Check sheet for the modelled part. Datum: model origin and axes. Units: mm. A direction names the side the tool comes from. Round coordinates to 2 decimals unless told otherwise and drop trailing zeros. Loops run counter-clockwise (first coordinate to the right, second up) from the corner with the lowest first, then second, coordinate; pieces in that order, holes last. Notation, with made-up numbers: (22, 86) - (64, 86) arc R32 cw to (64, 125) - close; hole circle Ø8 at (24.25, 84.5). An arc over 180 degrees is marked (long way). Put each result on its own line as item: value. Start each with the question number.
Autodesk Inventor part; units mm, degrees
ref_plane "YZ Plane" through (0, 0, 0) normal (1, 0, 0) x (0, 1, 0)
ref_plane "XZ Plane" through (0, 0, 0) normal (0, 1, 0) x (-1, 0, 0)
ref_plane "XY Plane" through (0, 0, 0) normal (0, 0, 1) x (1, 0, 0)
sketch "Sketch1" plane through (0, 0, 0) normal (0, 0, 1) x (1, 0, 0)
  line L0 (29.7558, 35.4616) -> (45.5886, 8.0385)
  line L1 (45.5886, 8.0385) -> (40.0899, -23.1459)
  line L2 (40.0899, -23.1459) -> (15.8328, -43.5001)
  line L3 (15.8328, -43.5001) -> (-15.8328, -43.5001)
  line L4 (-15.8328, -43.5001) -> (-40.0899, -23.1459)
  line L5 (-40.0899, -23.1459) -> (-45.5886, 8.0385)
  line L6 (-45.5886, 8.0385) -> (-29.7558, 35.4616)
  line L7 (-29.7558, 35.4616) -> (0, 46.2919)
  line L8 (0, 46.2919) -> (29.7558, 35.4616)
  line L9 (-29.7558, 35.4616) -> (0, 87.0003)
  line L10 (0, 87.0003) -> (29.7558, 35.4616)
  line L11 (0, 93.0003) -> (-48.7326, 8.5929)
  line L12 (-48.7326, 8.5929) -> (-42.8548, -24.7422)
  line L13 (-42.8548, -24.7422) -> (-16.9247, -46.5001)
  line L14 (-16.9247, -46.5001) -> (16.9247, -46.5001)
  line L15 (16.9247, -46.5001) -> (42.8548, -24.7422)
  line L16 (42.8548, -24.7422) -> (48.7326, 8.5929)
  line L17 (48.7326, 8.5929) -> (0, 93.0003)
  line L18 (0, -74.4002) -> (0, 120.9003)
  point P0 (0, 0)
  point P1 (0, 0)
  dimension "d0" = 89.792
  dimension "d1" = 3
  dimension "d2" = 3
  dimension "d3" = 3
  dimension "d4" = 3
extrude "Extrusion1" add sketch "Sketch1" along normal mid plane 20 contours L10 L18 L17 L16 L15 L14 L3 L2 L1 L0 | L9 L6 L5 L4 L3 L18 L14 L13 L12 L11
sketch "Sketch2" plane through (0, 0, 10) normal (0, 0, 1) x (1, 0, 0)
  line L0 (-1.5, 90.4022) -> (-1.5, 84.4022)
  line L1 (0, 87.0003) -> (-45.5886, 8.0385)
  line L2 (45.5886, 8.0385) -> (0, 87.0003)
  line L3 (1.5, 84.4022) -> (1.5, 90.4022)
  line L4 (48.7326, 8.5929) -> (0, 93.0003)
  line L5 (16.9247, -46.5001) -> (42.8548, -24.7422)
  line L6 (42.8548, -24.7422) -> (48.7326, 8.5929)
  line L7 (48.7326, 8.5929) -> (0, 93.0003)
  line L8 (0, 93.0003) -> (-48.7326, 8.5929)
  line L9 (-48.7326, 8.5929) -> (-42.8548, -24.7422)
  line L10 (-42.8548, -24.7422) -> (-16.9247, -46.5001)
  line L11 (-16.9247, -46.5001) -> (16.9247, -46.5001)
  line L12 (15.8328, -43.5001) -> (-15.8328, -43.5001)
  line L13 (-15.8328, -43.5001) -> (-40.0899, -23.1459)
  line L14 (-40.0899, -23.1459) -> (-45.5886, 8.0385)
  line L15 (-45.5886, 8.0385) -> (0, 87.0003)
  line L16 (0, 87.0003) -> (45.5886, 8.0385)
  line L17 (45.5886, 8.0385) -> (40.0899, -23.1459)
  line L18 (40.0899, -23.1459) -> (15.8328, -43.5001)
  line L19 (0, -74.4002) -> (0, 120.9003)
  point P0 (0, 0)
  dimension "d7" = 3
extrude "Extrusion2" cut sketch "Sketch2" against normal through all contours L8 L19 L1 L0 | L4 L3 L2 L19
sketch "Sketch3" plane through (0, 0, 0) normal (1, 0, 0) x (0, 1, 0)
  line L0 (90.4022, -10) -> (90.4022, 10)
  line L1 (8.5929, 10) -> (90.4022, 10)
  line L2 (8.5929, -10) -> (8.5929, 10)
  line L3 (90.4022, -10) -> (8.5929, -10)
  line L4 (55.4022, 6.5) -> (75.4022, 6.5)
  line L5 (75.4022, 6.5) -> (75.4022, -6.5)
  line L6 (75.4022, -6.5) -> (55.4022, -6.5)
  line L7 (55.4022, -6.5) -> (55.4022, 6.5)
  line L8 (55.4022, 6.5) -> (75.4022, -6.5) construction
  line L9 (75.4022, 6.5) -> (55.4022, -6.5) construction
  point P0 (0, 0)
  point P1 (65.4022, 0)
  point P2 (90.4022, 0)
  dimension "d10" = 13
  dimension "d11" = 15
  dimension "d12" = 20
extrude "Extrusion3" cut sketch "Sketch3" along normal through all both and the other way through all contours L4 L5 L6 L7
fillet "Fillet1" radius 3 8 edges at (8.4282, 75.4022, 6.5) (19.9752, 55.4022, 6.5) (19.9752, 55.4022, -6.5) (8.4282, 75.4022, -6.5) (-8.4282, 75.4022, -6.5) (-8.4282, 75.4022, 6.5) (-19.9752, 55.4022, 6.5) (-19.9752, 55.4022, -6.5)
sketch "Sketch5" plane through (0, 0, 10) normal (0, 0, 1) x (1, 0, 0)
  line L0 (1.5, 90.4022) -> (1.5, 84.4022)
  line L1 (1.5, 84.4022) -> (45.5886, 8.0385)
  line L2 (45.5886, 8.0385) -> (40.0899, -23.1459)
  line L3 (40.0899, -23.1459) -> (15.8328, -43.5001)
  line L4 (15.8328, -43.5001) -> (-15.8328, -43.5001)
  line L5 (-15.8328, -43.5001) -> (-40.0899, -23.1459)
  line L6 (-40.0899, -23.1459) -> (-45.5886, 8.0385)
  line L7 (-45.5886, 8.0385) -> (-1.5, 84.4022)
  line L8 (-1.5, 84.4022) -> (-1.5, 90.4022)
  line L9 (-1.5, 90.4022) -> (-48.7326, 8.5929)
  line L10 (-48.7326, 8.5929) -> (-42.8548, -24.7422)
  line L11 (-42.8548, -24.7422) -> (-16.9247, -46.5001)
  line L12 (-16.9247, -46.5001) -> (16.9247, -46.5001)
  line L13 (16.9247, -46.5001) -> (42.8548, -24.7422)
  line L14 (42.8548, -24.7422) -> (48.7326, 8.5929)
  line L15 (48.7326, 8.5929) -> (1.5, 90.4022)
  line L16 (-40.0899, -23.1459) -> (-42.8548, -24.7422)
  line L17 (40.0899, -23.1459) -> (45.5886, 8.0385)
  line L18 (40.0899, -23.1459) -> (42.8548, -24.7422)
  point P0 (0, 0)
extrude "Extrusion5" add sketch "Sketch5" along normal blind 2 contours L13 L12 L11 L16 L5 L4 L3 L18
sketch "Sketch6" plane through (0, 0, 12) normal (0, 0, 1) x (1, 0, 0)
  line L0 (15.8328, -43.5001) -> (-15.8328, -43.5001)
  line L1 (-15.8328, -43.5001) -> (-40.0899, -23.1459)
  line L2 (-40.0899, -23.1459) -> (-42.8548, -24.7422)
  line L3 (-42.8548, -24.7422) -> (-16.9247, -46.5001)
  line L4 (-16.9247, -46.5001) -> (16.9247, -46.5001)
  line L5 (16.9247, -46.5001) -> (42.8548, -24.7422)
  line L6 (42.8548, -24.7422) -> (40.0899, -23.1459)
  line L7 (40.0899, -23.1459) -> (15.8328, -43.5001)
  line L8 (-42.8548, -24.7422) -> (-36.4035, -21.0176)
  line L9 (-36.4035, -21.0176) -> (-14.3769, -39.5001)
  line L10 (-14.3769, -39.5001) -> (14.3769, -39.5001)
  line L11 (14.3769, -39.5001) -> (36.4035, -21.0176)
  line L12 (36.4035, -21.0176) -> (42.8548, -24.7422)
  line L13 (-40.0899, -23.1459) -> (-42.8548, -24.7422)
  line L14 (0, -73.8806) -> (0, 117.7826)
  point P0 (0, 0)
  dimension "d21" = 4
  dimension "d22" = 4
extrude "Extrusion6" add sketch "Sketch6" along normal blind 2
properties part number "HARNESS"
Q1. Cross-section at B-B on x = 33. Enter the section's corners in (y, z).
Q2. Depth check by flat-ended pin: pin 1 Ø6 at (y, z) = (-25.5, 9.5) entering from +X; pin 2 Ø11 at (x, z) = (1, 5) entering from +Y; pin 3 Ø9 at (x, y) = (13.5, 62.5) entering from +Z; pin 4 Ø6.5 at (y, z) = (88.5, -1.5) entering from -X. Enter the tip coordinate at first touch or a pass-through.
Q3. Material ranges on line 1 (Z direction, x = 44, y = -18); line 2 (X direction, y = -31, z = 1.5); line 3 (X direction, y = 76, z = -3.25), recorded low to high. Write a range as from..to.
Q4. Cross-section at A-A on z = -1.5. Enter the section's corners in (x, y), and give its area (3 significant figures).
Q5. Set-up check for faces 1 (the face through (-8, 75.402, 0)), 2 (the face through (0, -43.5, 1)), 3 (the face through (-20, 55.402, 0)): record each of +Z, -Z, +X, -X, +Y, -Y from which the full face is reachable in a straight line by a thin tool's end or side.
Q6. Cross-section at C-C on y = 6. Enter the section's corners in (x, z), and give its area (3 significant figures).
Q7. Cross-section at D-D on y = -32.5. Enter the section's corners in (x, z).
Q8. Draft check along Z on faces 4 (the face through (-33, 32, -10)), 5 (the face through (9.258, 74.5, 5.645)), 6 (the face through (-27.792, -33.465, 0.846)). Enter one of: +Z half, -Z half, draft (parallel to the pull), parting line (faces both ways), or undercut.
Answer list:
1. outline: (-33.01, -10) - (-29.1, -10) - (-29.1, 12) - (-23.87, 12) - (-23.87, 14) - (-33.01, 14) - close; (29.84, -10) - (35.84, -10) - (35.84, 10) - (29.84, 10) - close
2. pin 1: stops at x = 43.25
2. pin 2: stops at y = 90.4
2. pin 3: stops at z = 10
2. pin 4: stops at x = -4.47
3. line 1: z = -10..10
3. line 2: x = -35.4..-30.73, 30.73..35.4
3. line 3: x = -9.82..-6.35, 6.35..9.82
4. outline: (-48.73, 8.59) - (-42.85, -24.74) - (-16.92, -46.5) - (16.92, -46.5) - (42.85, -24.74) - (48.73, 8.59) - (21.71, 55.4) - (18.24, 55.4) - (29.76, 35.46) - (45.59, 8.04) - (40.09, -23.15) - (15.83, -43.5) - (-15.83, -43.5) - (-40.09, -23.15) - (-45.59, 8.04) - (-29.76, 35.46) - (-18.24, 55.4) - (-21.71, 55.4) - close; (-10.16, 75.4) - (-6.7, 75.4) - (-1.5, 84.4) - (-1.5, 90.4) - close; (1.5, 84.4) - (6.7, 75.4) - (10.16, 75.4) - (1.5, 90.4) - close
4. area: 901 mm2
5. face 1: +X, -X
5. face 2: -Z
5. face 3: +X, -X, +Y
6. outline: (-48.28, -10) - (-45.23, -10) - (-45.23, 10) - (-48.28, 10) - close; (45.23, -10) - (48.28, -10) - (48.28, 10) - (45.23, 10) - close
6. area: 122 mm2
7. outline: (-33.61, -10) - (-28.94, -10) - (-28.94, 12) - (-22.72, 12) - (-22.72, 14) - (-33.61, 14) - close; (22.72, 12) - (28.94, 12) - (28.94, -10) - (33.61, -10) - (33.61, 14) - (22.72, 14) - close
8. face 4: -Z half
8. face 5: undercut
8. face 6: draft
